```python
from build123d import *

# Parameters (mm, degrees)
BOSS_EXTRUDE1_DEPTH = 3
SKETCH2_W           = 15
SKETCH2_H           = 3
BOSS_EXTRUDE2_DEPTH = 4
SKETCH3_R           = 1.4732
CUT_EXTRUDE1_DEPTH  = 4


with BuildPart() as part:
    # Sketch1 → Boss-Extrude1 (new body)
    with BuildSketch(Plane(origin=(0, 0, 0), x_dir=(1, 0, 0), z_dir=(0, 1, 0))):
        Polygon((-48.209070726, -57.453333234), (0, 75), (0, 0), align=None)
    extrude(amount=BOSS_EXTRUDE1_DEPTH)

    # Sketch2 → Boss-Extrude2 (add)
    with BuildSketch(Plane(origin=(0, 0, 0), x_dir=(0, 0, -1), z_dir=(1, 0, 0))):
        with Locations((7.5, 1.5)):
            Rectangle(SKETCH2_W, SKETCH2_H)
        with Locations((67.5, 1.5)):
            Rectangle(SKETCH2_W, SKETCH2_H)
    extrude(amount=BOSS_EXTRUDE2_DEPTH)

    # Sketch3 → Cut-Extrude1 (cut, through all)
    with BuildSketch(Plane(origin=(0, 3, 0), x_dir=(1, 0, 0), z_dir=(0, 1, 0))):
        with Locations((-2.5, 37.5)):
            Circle(SKETCH3_R)
    extrude(amount=-CUT_EXTRUDE1_DEPTH, mode=Mode.SUBTRACT)


solid = part.part
```
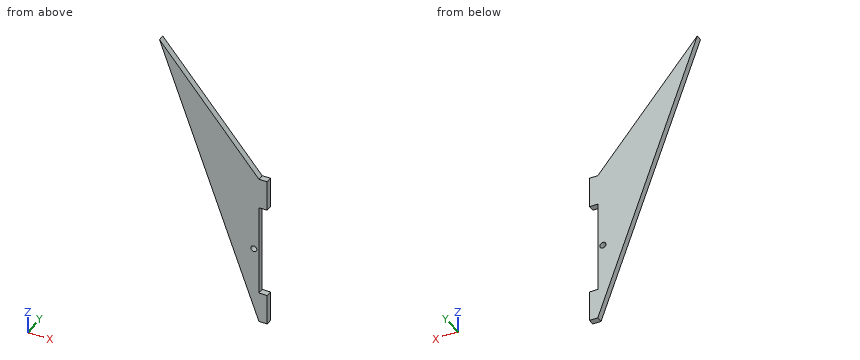
Can you work these out from the model? Positions are in its coordinate system, mm. Coordinates: 2 decimals unless noted, no trailing zeros. Order: outer loops, then holes, each group sorted by start corner. A loop starts at its lowest first (then second) coordinate and runs counter-clockwise, first axis right, second up. Notation, with made-up numbers: (-7.75, 18.25) - (20.25, 18.25) arc R16 cw to (20.25, 48.25) - close; hole circle Ø9 at (24.5, 16). An arc over 180 degrees is marked (long way). Answer in a Markdown table with one row per item.
1. Suppose I cut it at A-A (y = 2.55). Please give me the cut outline in (x, z).
Reply:
| item | result |
|---|---|
| outline | (-48.21, 57.45) - (0, -75) - (4, -75) - (4, -60) - (0, -60) - (0, -15) - (4, -15) - (4, 0) - (0, 0) - close; hole circle Ø2.95 at (-2.5, -37.5) |
2. Suppose I cut it at D-D (z = 26.5). Please give me the cut outline in (x, y), and give its area (3 significant figures).
Reply:
| item | result |
|---|---|
| outline | (-36.94, 0) - (-22.24, 0) - (-22.24, 3) - (-36.94, 3) - close |
| area | 44.1 mm^2 |
3. Suppose I cut it at B-B (z = -37.5). Please give me the cut outline in (x, y).
Reply:
| item | result |
|---|---|
| outline | (-13.65, 0) - (-3.97, 0) - (-3.97, 3) - (-13.65, 3) - close; (-1.03, 0) - (0, 0) - (0, 3) - (-1.03, 3) - close |
4. For pin 1 (3 mm diameter, centred on x = -11.5, z = -39, fed in from -Y), with a flat end and sliding along its axis, tell me the tip position at first contact or that it passes through.
Reply:
| item | result |
|---|---|
| pin 1 | stops at y = 0 |
5. If I drill on line 1 along Z through (x, y) = (1, 1.9); line 2 along X through (y, z) = (1.35, -37.5); line 3 along X through (y, z) = (0.55, -46.5), over which ranges is the centre line in solid material (lowest first)?
Reply:
| item | result |
|---|---|
| line 1 | z = -75 to -60, -15 to 0 |
| line 2 | x = -13.65 to -3.97, -1.03 to 0 |
| line 3 | x = -10.37 to 0 |
6. Suppose I cut it at C-C (x = -2.5). Please give me the cut outline in (y, z).
Reply:
| item | result |
|---|---|
| outline | (0, -68.13) - (3, -68.13) - (3, -38.97) - (0, -38.97) - close; (0, -36.03) - (3, -36.03) - (3, 2.98) - (0, 2.98) - close |
